For this review, take the finished solid that the model builds, in its own axes (mm). A direction names the side the tool comes from. Give positions to 0.01 mm unless a question says otherwise; leave off trailing zeros. Write each loop counter-clockwise with the first axis right and the second up, starting at its lowest first coordinate (ties: lowest second). Pieces come first, ordered by that corner, then holes. Notation, with made-up numbers: M 78,26.25 L 97,26.25 A25 cw 97,44.25 Z; hole C 51.25,59.25 d4. An arc over 180 degrees is marked long. Answer as a JSON object with one key per item and string values. Group by question number.
```python
from build123d import *

# Parameters (mm, degrees)
MODEL_R             = 0.5
BOSS_EXTRUDE1_DEPTH = 1


with BuildPart() as part:
    # Model → Boss-Extrude1 (new body)
    with BuildSketch(Plane.XY):
        with BuildLine():
            Line((82.651854623, -0.999998655), (54.651854623, -0.999998655))
            ThreePointArc((54.651854623, -0.999998655), (53.944747842, -0.707105436), (53.651854623, 1.345e-06))
            Line((53.651854623, 1.345e-06), (53.651854623, 73.585787783))
            ThreePointArc((53.651854623, 73.585787783), (54.26917119, 74.509667315), (55.358961404, 74.292894564))
            Line((55.358961404, 74.292894564), (59.148961404, 70.502894564))
            ThreePointArc((59.148961404, 70.502894564), (59.365734155, 70.178471215), (59.441854623, 69.795787783))
            Line((59.441854623, 69.795787783), (59.441854623, 18.780001734))
            Line((59.441854623, 18.780001734), (61.441849513, 16.780001345))
            Line((61.441849513, 16.780001345), (75.861849513, 16.780001345))
            Line((75.861849513, 16.780001345), (77.861854623, 18.780001734))
            Line((77.861854623, 18.780001734), (77.861854623, 69.795787783))
            ThreePointArc((77.861854623, 69.795787783), (77.93797509, 70.178471215), (78.154747842, 70.502894564))
            Line((78.154747842, 70.502894564), (81.944747842, 74.292894564))
            ThreePointArc((81.944747842, 74.292894564), (83.034538055, 74.509667315), (83.651854623, 73.585787783))
            Line((83.651854623, 73.585787783), (83.651854623, 1.345e-06))
            ThreePointArc((83.651854623, 1.345e-06), (83.358961404, -0.707105436), (82.651854623, -0.999998655))
        make_face()
        with Locations((56.151854623, 6.500001345)):
            Circle(MODEL_R, mode=Mode.SUBTRACT)
        with Locations((56.151854623, 71.500001345)):
            Circle(MODEL_R, mode=Mode.SUBTRACT)
        with Locations((81.151854623, 6.500001345)):
            Circle(MODEL_R, mode=Mode.SUBTRACT)
        with Locations((81.151854623, 71.500001345)):
            Circle(MODEL_R, mode=Mode.SUBTRACT)
        with Locations((56.151854623, 1.500001345)):
            Circle(MODEL_R, mode=Mode.SUBTRACT)
        with Locations((81.151854623, 1.500001345)):
            Circle(MODEL_R, mode=Mode.SUBTRACT)
    extrude(amount=BOSS_EXTRUDE1_DEPTH)


solid = part.part
```
Item 1: Consider section A-A (y = 19.5). Give the boundary of the cut face in (x, z).
Item 2: Consider section C-C (x = 73.5). Give the boundary of the cut face in (y, z).
Item 3: Insertion check: P1, Ø8, axis at x = 71.5, y = 36.5, coming from the +Z side. The pin has a flat end and moves straight along its axis. Give the tip position at first contact, or say it passes through.
Item 4: Consider section B-B (z = 0.75). Give the boundary of the cut face in (x, y).
Item 5: Machinability: for faces 1 (the flat face through (79, 29, 0)), 2 (the flat face through (60.43, 17.79, 0.49)), which of the approach directions +Z, -Z, +X, -X, +Y, -Y give a long, thin tool a straight path to every point of the face, cutting with its end or side? Answer none if there is none.
Item 6: To check wall thickness, follow probe 1 along X at (y, z) = (41.5, 0.25); probe 2 along Y at (x, z) = (81.5, 0.95); probe 3 along Y at (x, z) = (72, 0.7). State the ranges of each line that lie inside material, in increasing order.
Item 7: Consider section D-D (x = 80). Give the boundary of the cut face in (y, z).
Result set:
{
 "1": {"outline": "M 53.65,0 L 59.44,0 L 59.44,1 L 53.65,1 Z; M 77.86,0 L 83.65,0 L 83.65,1 L 77.86,1 Z"},
 "2": {"outline": "M -1,0 L 16.78,0 L 16.78,1 L -1,1 Z"},
 "3": {"P1": "passes through"},
 "4": {"outline": "M 53.65,0 A1 ccw 54.65,-1 L 82.65,-1 A1 ccw 83.65,0 L 83.65,73.59 A1 ccw 81.94,74.29 L 78.15,70.5 A1 ccw 77.86,69.8 L 77.86,18.78 L 75.86,16.78 L 61.44,16.78 L 59.44,18.78 L 59.44,69.8 A1 ccw 59.15,70.5 L 55.36,74.29 A1 ccw 53.65,73.59 Z; hole C 56.15,1.5 d1; hole C 56.15,6.5 d1; hole C 56.15,71.5 d1; hole C 81.15,1.5 d1; hole C 81.15,6.5 d1; hole C 81.15,71.5 d1"},
 "5": {"face 1": "-Z, +X, -X, +Y, -Y", "face 2": "+Z, -Z, +Y"},
 "6": {"probe 1": "x = 53.65 to 59.44, 77.86 to 83.65", "probe 2": "y = -1 to 1.14, 1.86 to 6.14, 6.86 to 71.14, 71.86 to 73.85", "probe 3": "y = -1 to 16.78"},
 "7": {"outline": "M -1,0 L 72.35,0 L 72.35,1 L -1,1 Z"}
}
